Design review of the part built by this model. Coordinates are the model's own, in mm. A direction names the side the tool comes from. Give positions to 0.01 mm unless a question says otherwise; leave off trailing zeros. Write each loop counter-clockwise with the first axis right and the second up, starting at its lowest first coordinate (ties: lowest second). Pieces come first, ordered by that corner, then holes. Notation, with made-up numbers: M 88.5,-4.5 L 92.5,-4.5 A14 ccw 92.5,4.5 Z; hole C -34,-23.75 d11. An arc over 180 degrees is marked long. Use a Markdown table: item, result. Add a question column.
```python
from build123d import *

# Parameters (mm, degrees)
CYLINDER_R     = 7
CYLINDER_DEPTH = 2.5
CHAMFER_SIZE   = 0.6
ARRAY_COUNT    = 7
FILLET_R       = 1.5
POCKET_DEPTH   = 5


with BuildPart() as chamfer_body:
    # Cylinder → Cylinder (new body)
    with BuildSketch(Plane.XY.offset(-2.5)):
        Circle(CYLINDER_R)
    extrude(amount=CYLINDER_DEPTH)

    # Chamfer
    chamfer_edges = [chamfer_body.edges().sort_by_distance(p)[0] for p in [
        (-7, 0, 0),
    ]]
    chamfer(chamfer_edges, length=CHAMFER_SIZE)


with BuildPart() as array:
    # Cone001 → Cone001 (revolve)
    with BuildSketch(Plane(origin=(0, 5.3, -1), x_dir=(1, 0, 0), z_dir=(0, -1, 0))):
        Polygon((0, 0), (0.8, 0), (1.5, 10), (0, 10), align=None)
    revolve(axis=Axis((0, 5.3, -1), (0, 0, 1)))

    # Array: Array ×7 about axis
    array_axis = Axis((0, 0, 0), (0, 0, 1))


with BuildPart() as array_1:
    add(array.part)
    for i in range(1, ARRAY_COUNT):
        add(array.part.rotate(array_axis, i * 360 / ARRAY_COUNT))


with BuildPart() as pocket:
    # Cone → Cone (revolve)
    with BuildSketch(Plane.XZ):
        Polygon((0, 0), (5, 0), (4.5, 8), (0, 8), align=None)
    revolve(axis=Axis((0, 0, 0), (0, 0, 1)))

    # Fillet
    fillet_edges = [pocket.edges().sort_by_distance(p)[0] for p in [
        (-4.5, 0, 8),
    ]]
    fillet(fillet_edges, radius=FILLET_R)

    # Cut: cut Array
    add(array_1.part, mode=Mode.SUBTRACT)

    # Fusion: union Chamfer body
    add(chamfer_body.part)

    # Sketch → Pocket (cut)
    with BuildSketch(Plane(origin=(0, 0, -2.5), x_dir=(1, 0, 0), z_dir=(0, 0, -1))):
        with BuildLine():
            ThreePointArc((2, 1.5), (-2.5, 0), (2, -1.5))
            Line((2, 1.5), (2, -1.5))
        make_face()
    extrude(amount=-POCKET_DEPTH, mode=Mode.SUBTRACT)


solid = pocket.part
```
(1) Wall thickness on L1, parallel to Y at x = 0, z = -1.15; L2, parallel to Z at x = 1.75, y = -4.5; L3, parallel to X at y = -1.75, z = 2.25: over which ranges is each line inside the solid? List them lowest first.
(2) For pin 1 (2 mm diameter, centred on x = -4.5, z = 0, fed in from +Y); pin 2 (1.5 mm diameter, centred on y = -1.5, z = 6, fed in from -X); pin 3 (2 mm diameter, centred on x = 1, z = 0.5, fed in from +Y), all flat-tipped, find the tip position at first contact; note any pin that passes through.
(3) Machinability: for faces 1 (the flat face through (2, 0, 0)), 2 (the conical face through (-0.018, 4.154, 3.94)), 3 (the flat face through (1.9, -4.2, 0)), which of the approach directions +Z, -Z, +X, -X, +Y, -Y give a long, thin tool a straight path to every point of the face, cutting with its end or side? Answer none if there is none.
(4) The part is to be moulded in two halves that separate along Y. For faces 4 (the conical face through (-3.76, -2.97, 3.34)), 5 (the flat face through (0, 0, 8)), 6 (the conical face through (3.24, 2.6, 3.94)), say which applies: released by +Y, released by -Y, zero draft, split by the parting line, or undercut.
(5) Add section A-A on x = 0. Give the boundary of the cut face in (y, z), then the cut area to 3 significant figures.
(6) Add section B-B on z = -1.5. Give the boundary of the cut face in (x, y), then the cut area to 3 significant figures.
From the geometry:
| question | item | result |
|---|---|---|
| 1 | L1 | y = -7 to -2.5, 2.5 to 7 |
| 1 | L2 | z = -2.5 to 0 |
| 1 | L3 | x = -4.31 to -1.79, 1.79 to 4.31 |
| 2 | pin 1 | stops at y = 5.94 |
| 2 | pin 2 | stops at x = -4.21 |
| 2 | pin 3 | stops at y = 6.84 |
| 3 | face 1 | -Z |
| 3 | face 2 | +Z, +Y |
| 3 | face 3 | +Z |
| 4 | face 4 | released by -Y |
| 4 | face 5 | zero draft |
| 4 | face 6 | undercut |
| 5 | outline | M -7,-2.5 L -2.5,-2.5 L -2.5,2.5 L 2.5,2.5 L 2.5,-2.5 L 7,-2.5 L 7,-0.6 L 6.4,0 L 4.43,0 L 3.89,7.77 A1.5 ccw 3.09,8 L -3.09,8 A1.5 ccw -4.59,6.59 L -5,0 L -6.4,0 L -7,-0.6 Z |
| 5 | area | 80.4 mm^2 |
| 6 | outline | C 0,0 d14; hole M 2,-1.5 L 2,1.5 A2.5 ccw long Z |
| 6 | area | 135 mm^2 |
